from build123d import *

# Parameters (mm, degrees)
BOSS_EXTRUDE1_DEPTH = 90
SKETCH2_R           = 1.9
CUT_EXTRUDE1_DEPTH  = 99.020406039
SKETCH3_W           = 8
SKETCH3_H           = 4
CUT_EXTRUDE2_DEPTH  = 97.503885932


with BuildPart() as part:
    # Sketch1 → Boss-Extrude1 (new body)
    with BuildSketch(Plane.XY):
        Polygon((11, 5), (-11, 5), (-11, -5), (-16, -5), (-16, -22), (-6, -22), (-6, -17), (-11, -17), (-11, -10), (11, -10), (11, -17), (6, -17), (6, -22), (16, -22), (16, -5), (11, -5), align=None)
    extrude(amount=-BOSS_EXTRUDE1_DEPTH)

    # Sketch2 → Cut-Extrude1 (cut, through all)
    with BuildSketch(Plane(origin=(16, 0, 0), x_dir=(0, 0, -1), z_dir=(1, 0, 0))):
        with Locations((45, -13.5)):
            Circle(SKETCH2_R)
        with Locations((62, -13.5)):
            Circle(SKETCH2_R)
        with Locations((79, -13.5)):
            Circle(SKETCH2_R)
        with Locations((28, -13.5)):
            Circle(SKETCH2_R)
        with Locations((11, -13.5)):
            Circle(SKETCH2_R)
    extrude(amount=-CUT_EXTRUDE1_DEPTH, mode=Mode.SUBTRACT)

    # Sketch3 → Cut-Extrude2 (cut, through all)
    with BuildSketch(Plane(origin=(11, 0, 0), x_dir=(0, 0, -1), z_dir=(1, 0, 0))):
        with Locations((62, 0)):
            Rectangle(SKETCH3_W, SKETCH3_H)
        with Locations((45, 0)):
            Rectangle(SKETCH3_W, SKETCH3_H)
        with Locations((79, 0)):
            Rectangle(SKETCH3_W, SKETCH3_H)
        with Locations((28, 0)):
            Rectangle(SKETCH3_W, SKETCH3_H)
        with Locations((11, 0)):
            Rectangle(SKETCH3_W, SKETCH3_H)
    extrude(amount=-CUT_EXTRUDE2_DEPTH, mode=Mode.SUBTRACT)


solid = part.part
The model under review builds one solid part; all positions refer to its coordinate system, in mm. A direction names the side the tool comes from. Round coordinates to 2 decimals unless told otherwise and drop trailing zeros. Loops run counter-clockwise (first coordinate to the right, second up) from the corner with the lowest first, then second, coordinate; pieces in that order, holes last. Notation, with made-up numbers: M -34.5,-10.75 L -26.5,-10.75 A29 cw -26.5,25.25 Z; hole C 67.25,34 d11. An arc over 180 degrees is marked long. Answer as CSV lines item,"result". Start each with the question number.
Item 1: Consider section C-C (z = -62). Write out the cut boundary in (x, y), then the cut area to 3 significant figures.
Item 2: Mouldability with a two-part tool opening along Y and no side actions: class faces 4 (the face through (0, 0, -66)), 5 (the face through (0, 5, -44)), 6 (the face through (11, -22, -44)) as released by +Y, released by -Y, zero draft, split by the parting line, or undercut.
Item 3: Insertion check: P1, Ø4.5, axis at x = 3.5, y = 0, coming from the +Z side; P2, Ø2.5, axis at x = 14, z = -66, coming from the +Y side; P3, Ø4, axis at x = -3, z = -28.5, coming from the -Y side; P4, Ø2, axis at y = 0.5, z = -74, coming from the -X side. Each pin has a flat end and moves straight along its axis. Give the tip position at first contact, or say it passes through.
Item 4: Consider section D-D (y = -13.5). State how many separate pieces and enclosed holes the cut face has, then the cut area to 3 significant figures.
Item 5: Wall thickness on line 1 (Z direction, x = 7, y = -1.75); line 2 (Y direction, x = 13, z = -45); line 3 (X direction, y = -10.25, z = -67): over which ranges is each line inside the solid? List them lowest first. Write a range as [from, to].
Item 6: Consider section B-B (y = -20). Write out the cut boundary in (x, z), then the cut area to 3 significant figures.
Item 7: Consider section A-A (x = -3). Write out the cut boundary in (y, z), then the cut area to 3 significant figures.
Item 8: For faces 1 (the face through (0, 2, -11)), 2 (the face through (-13, -5, -44)), 3 (the face through (11, -11, -44)), list the 3-axis set-ups (+Z, -Z, +X, -X, +Y, -Y) from which the entire face can be reached by the end or side of a thin tool; tool diameter is ignored.
Answer:
1,outline,"M -16,-22 L -6,-22 L -6,-17 L -11,-17 L -11,-15.4 L -16,-15.4 Z; M -16,-11.6 L -11,-11.6 L -11,-10 L 11,-10 L 11,-11.6 L 16,-11.6 L 16,-5 L 11,-5 L 11,-2 L -11,-2 L -11,-5 L -16,-5 Z; M -11,2 L 11,2 L 11,5 L -11,5 Z; M 6,-22 L 16,-22 L 16,-15.4 L 11,-15.4 L 11,-17 L 6,-17 Z"
1,area,"424 mm^2"
2,face 4,"undercut"
2,face 5,"released by +Y"
2,face 6,"released by -Y"
3,P1,"stops at z = 0"
3,P2,"stops at y = -5"
3,P3,"stops at y = -10"
3,P4,"stops at x = -11"
4,separate pieces,"12"
4,enclosed holes,"0"
4,area,"710 mm^2"
5,line 1,"z = [-90, -83], [-75, -66], [-58, -49], [-41, -32], [-24, -15], [-7, 0]"
5,line 2,"y = [-22, -15.4], [-11.6, -5]"
5,line 3,"x = [-16, -11], [11, 16]"
6,outline,"M -16,-90 L -6,-90 L -6,0 L -16,0 Z; M 6,-90 L 16,-90 L 16,0 L 6,0 Z"
6,area,"1,800 mm^2"
7,outline,"M -10,-90 L 5,-90 L 5,0 L -10,0 Z; hole M -2,-83 L 2,-83 L 2,-75 L -2,-75 Z; hole M -2,-66 L 2,-66 L 2,-58 L -2,-58 Z; hole M -2,-49 L 2,-49 L 2,-41 L -2,-41 Z; hole M -2,-32 L 2,-32 L 2,-24 L -2,-24 Z; hole M -2,-15 L 2,-15 L 2,-7 L -2,-7 Z"
7,area,"1,190 mm^2"
8,face 1,"+X, -X"
8,face 2,"+Z, -Z, -X, +Y"
8,face 3,"+Z, -Z"
